Can you work these out from the model? Positions are in its coordinate system, mm. Face numbers are marked on the shaded views. Give positions to 0.01 mm unless a question says otherwise; leave off trailing zeros. Loops run counter-clockwise (first coordinate to the right, second up) from the corner with the lowest first, then second, coordinate; pieces in that order, holes last. Notation, with made-up numbers: (7, 88.25) - (58, 88.25) arc R18 ccw to (58, 99.25) - close; hole circle Ø5 at (79, 16). An arc over 180 degrees is marked (long way). Answer as a JSON object with one key per item and string values. Group by question number.
Item 1: Suppose I cut it at C-C on x = 39. Write out the boundary of the cut face in (y, z), and give its area (3 significant figures).
Item 2: Please list where these lines run through material, in increasing order: L1, parallel to X at y = 1.35, z = -30.5; L2, parallel to Z at x = 5, y = 1.8; L3, parallel to Z at x = 26, y = 0.3.
Item 3: Suppose I cut it at D-D on z = -19. Write out the boundary of the cut face in (x, y).
Item 4: Suppose I cut it at A-A on z = -37.5. Write out the boundary of the cut face in (x, y).
Item 5: Will these pins go through, and if not, where does the flat tip stop? pin 1 (1.3 mm diameter, centred on x = 2.5, z = -31.5, fed in from +Y); pin 2 (5.5 mm diameter, centred on x = 26.5, z = -38.5, fed in from +Y); pin 3 (2 mm diameter, centred on y = 1.5, z = -4, fed in from -X); pin 4 (5.5 mm diameter, centred on x = 36, z = -9, fed in from +Y).
Item 6: Thinking about a two-plate mould opening in Z: for the marked faces 1, 2 and 3, which applies, pulls with the +Z half, pulls with the -Z half, needs draft (parallel to the pull), parting line crosses it, or undercut?
Item 7: Suppose I cut it at B-B on x = 5. Write out the boundary of the cut face in (y, z), and give its area (3 significant figures).
from build123d import *

# Parameters (mm, degrees)
SKETCH1_W                                           = 53
SKETCH1_H                                           = 34
BOSS_EXTRUDE1_DEPTH                                 = 4
SKETCH2_W                                           = 8
SKETCH2_H                                           = 7
BOSS_EXTRUDE2_DEPTH                                 = 2.5
SKETCH3_W                                           = 48.6
SKETCH3_H                                           = 31.6
CUT_EXTRUDE1_DEPTH                                  = 3
SKETCH4_W                                           = 5.8
SKETCH4_H                                           = 4.3
SKETCH4_H_2                                         = 5.8
BOSS_EXTRUDE3_DEPTH                                 = 1
CUT_EXTRUDE2_DEPTH                                  = 1
SKETCH6_W                                           = 1.2
SKETCH6_H                                           = 10
SKETCH6_W_2                                         = 3.2
SKETCH6_H_2                                         = 30.4
CUT_EXTRUDE3_DEPTH                                  = 0.5
CSK_FOR_M3_COUNTERSUNK_FLAT_HEAD_SCR_2_COUNT        = 2
CSK_FOR_M3_COUNTERSUNK_FLAT_HEAD_SCR_2_PITCH        = 41
CSK_FOR_M2_COUNTERSUNK_FLAT_HEAD_SCREW1_D           = 2.4
CSK_FOR_M2_COUNTERSUNK_FLAT_HEAD_SCREW1_CSINK_D     = 4.4
CSK_FOR_M2_COUNTERSUNK_FLAT_HEAD_SCREW1_CSINK_ANGLE = 90


with BuildPart() as part:
    # Sketch1 → Boss-Extrude1 (new body)
    with BuildSketch(Plane(origin=(0, 0, 0), x_dir=(1, 0, 0), z_dir=(0, 1, 0))):
        with Locations((26.5, 17)):
            Rectangle(SKETCH1_W, SKETCH1_H)
    extrude(amount=BOSS_EXTRUDE1_DEPTH)

    # Sketch2 → Boss-Extrude2 (add)
    with BuildSketch(Plane(origin=(0, 0, 0), x_dir=(1, 0, 0), z_dir=(0, 1, 0))):
        with Locations((26, -3.5)):
            Rectangle(SKETCH2_W, SKETCH2_H)
        with Locations((26, 37.5)):
            Rectangle(SKETCH2_W, SKETCH2_H)
    extrude(amount=BOSS_EXTRUDE2_DEPTH)

    # Sketch3 → Cut-Extrude1 (cut)
    with BuildSketch(Plane(origin=(0, 4, 0), x_dir=(1, 0, 0), z_dir=(0, 1, 0))):
        with Locations((25.5, 17)):
            Rectangle(SKETCH3_W, SKETCH3_H)
    extrude(amount=-CUT_EXTRUDE1_DEPTH, mode=Mode.SUBTRACT)

    # Sketch4 → Boss-Extrude3 (add)
    with BuildSketch(Plane(origin=(0, 1, 0), x_dir=(1, 0, 0), z_dir=(0, 1, 0))):
        with Locations((4.1, 30.65)):
            Rectangle(SKETCH4_W, SKETCH4_H)
        with Locations((4.1, 4.1)):
            Rectangle(SKETCH4_W, SKETCH4_H_2)
    extrude(amount=BOSS_EXTRUDE3_DEPTH)

    # Sketch5 → Cut-Extrude2 (cut)
    with BuildSketch(Plane(origin=(0, 4, 0), x_dir=(1, 0, 0), z_dir=(0, 1, 0))):
        Polygon((49.8, 32.8), (1.2, 32.8), (1.2, 22), (0.8, 22), (0.8, 33.2), (49.8, 33.2), align=None)
        Polygon((49.8, 1.2), (1.2, 1.2), (1.2, 12), (0.8, 12), (0.8, 0.8), (49.8, 0.8), align=None)
    extrude(amount=-CUT_EXTRUDE2_DEPTH, mode=Mode.SUBTRACT)

    # Sketch6 → Cut-Extrude3 (cut)
    with BuildSketch(Plane(origin=(0, 4, 0), x_dir=(1, 0, 0), z_dir=(0, 1, 0))):
        with Locations((0.6, 17)):
            Rectangle(SKETCH6_W, SKETCH6_H)
        with Locations((51.4, 17)):
            Rectangle(SKETCH6_W_2, SKETCH6_H_2)
    extrude(amount=-CUT_EXTRUDE3_DEPTH, mode=Mode.SUBTRACT)

    # Sketch8 → CSK for M3 Countersunk Flat Head Screw1 (revolve, cut)
    with BuildSketch(Plane(origin=(26, 2.5, -37.5), x_dir=(0, 0, 1), z_dir=(1, 0, 0))):
        Polygon((0, 0), (0, 2.5), (1.7, 2.5), (1.7, 1.45), (3.15, 0), align=None)
    csk_for_m3_countersunk_flat_head_screw1 = revolve(axis=Axis((26, 8.85, -37.5), (0, -1, 0)), mode=Mode.SUBTRACT)

    # CSK for M3 Countersunk Flat Head Scr 2: CSK for M3 Countersunk Flat Head Screw1 ×2
    with Locations(*[(0, 0, i * CSK_FOR_M3_COUNTERSUNK_FLAT_HEAD_SCR_2_PITCH) for i in range(1, CSK_FOR_M3_COUNTERSUNK_FLAT_HEAD_SCR_2_COUNT)]):
        add(csk_for_m3_countersunk_flat_head_screw1, mode=Mode.SUBTRACT)

    # CSK for M2 Countersunk Flat Head Screw1 (through all)
    with Locations(Plane(origin=(5, 0, -5), x_dir=(0, 0, -1), z_dir=(0, -1, 0))):
        with Locations((0, 0), (25.5, 0)):
            CounterSinkHole(CSK_FOR_M2_COUNTERSUNK_FLAT_HEAD_SCREW1_D / 2, CSK_FOR_M2_COUNTERSUNK_FLAT_HEAD_SCREW1_CSINK_D / 2, counter_sink_angle=CSK_FOR_M2_COUNTERSUNK_FLAT_HEAD_SCREW1_CSINK_ANGLE)


solid = part.part
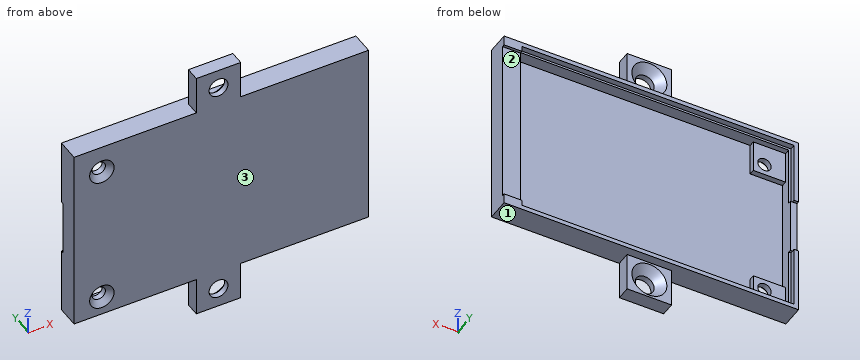
Worked out:
{
 "1": {"outline": "(0, -34) - (4, -34) - (4, -33.2) - (3, -33.2) - (3, -32.8) - (1, -32.8) - (1, -1.2) - (3, -1.2) - (3, -0.8) - (4, -0.8) - (4, 0) - (0, 0) - close", "area": "40.4 mm2"},
 "2": {"L1": "x = 0 to 3.8, 6.2 to 7, 49.8 to 53", "L2": "z = -34 to -31.7, -29.3 to -28.5, -7 to -6.2, -3.8 to 0", "L3": "z = -41 to -39.2, -35.8 to 1.8, 5.2 to 7"},
 "3": {"outline": "(0, 0) - (53, 0) - (53, 3.5) - (49.8, 3.5) - (49.8, 1) - (1.2, 1) - (1.2, 3.5) - (0, 3.5) - close"},
 "4": {"outline": "(22, 0) - (24.3, 0) - (24.3, 1.05) - (22.85, 2.5) - (22, 2.5) - close; (27.7, 0) - (30, 0) - (30, 2.5) - (29.15, 2.5) - (27.7, 1.05) - close"},
 "5": {"pin 1": "stops at y = 2", "pin 2": "stops at y = 2.5", "pin 3": "stops at x = 0", "pin 4": "stops at y = 1"},
 "6": {"face 1": "pulls with the -Z half", "face 2": "undercut", "face 3": "needs draft"},
 "7": {"outline": "(0, -34) - (4, -34) - (4, -33.2) - (3, -33.2) - (3, -32.8) - (2, -32.8) - (2, -31.7) - (1, -31.7) - (0, -32.7) - close; (0, -28.3) - (1, -29.3) - (2, -29.3) - (2, -28.5) - (1, -28.5) - (1, -7) - (2, -7) - (2, -6.2) - (1, -6.2) - (0, -7.2) - close; (0, -2.8) - (1, -3.8) - (2, -3.8) - (2, -1.2) - (3, -1.2) - (3, -0.8) - (4, -0.8) - (4, 0) - (0, 0) - close", "area": "38.9 mm2"}
}
